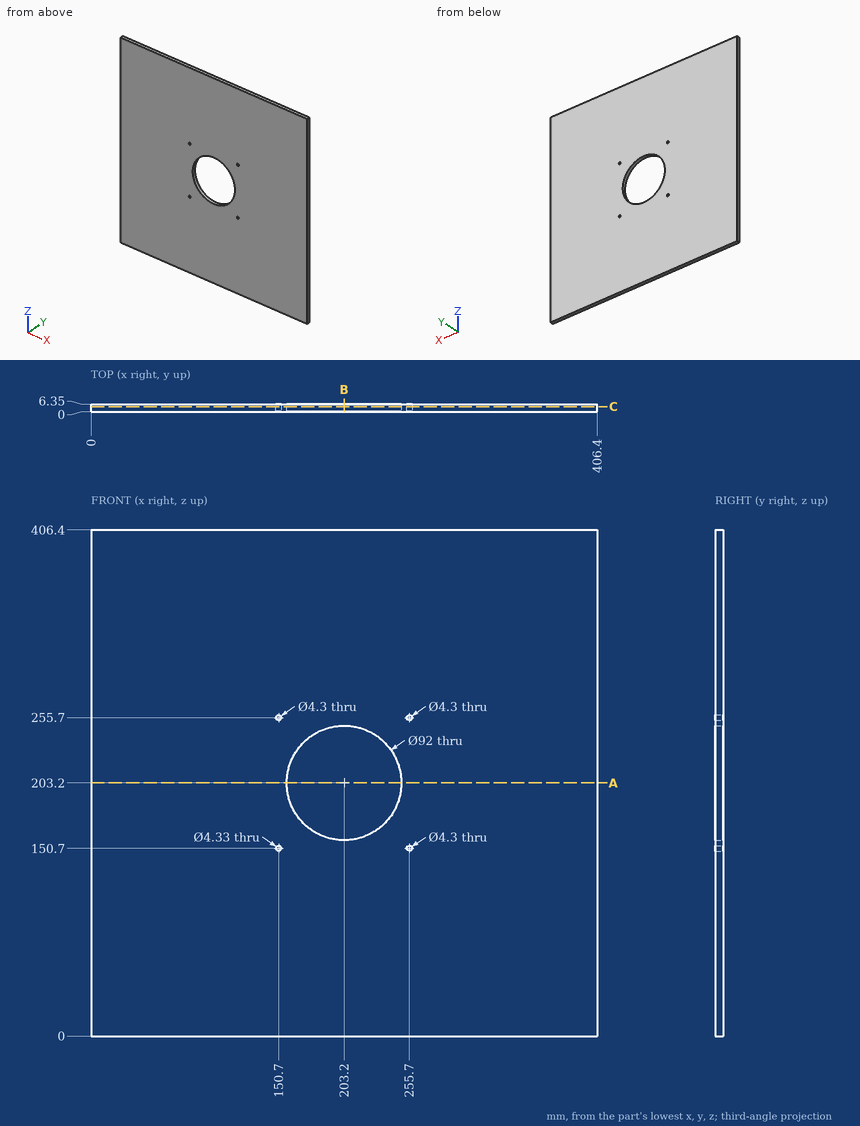
Input: dimensioned drawing with shaded views. Units: mm. Origin: part minimum x, y, z. Give positions to 0.01 mm unless a question says otherwise; leave off trailing zeros. Write each loop counter-clockwise with the first axis right and the second up, starting at its lowest first coordinate (ties: lowest second). Pieces come first, ordered by that corner, then holes. Notation, with made-up numbers: (56.25, -14.75) - (73.25, -14.75) arc R15 ccw to (73.25, 4.25) - close; hole circle Ø5 at (-19, -7). An arc over 180 degrees is marked (long way). One line per item, written item: value. Start each with the question number.
Q1. First-contact query: pin 1 Ø7 at (x, z) = (150.7, 255.7) entering from +Y. Flat tip, straight axial feed; report the tip coordinate or a pass-through.
Q2. Section query C-C, the plane y = 4.25. Return the cut outline in (x, z) (3 decimals), then the cut area to 3 significant figures.
Q3. Section query B-B, the plane x = 203.2. Return the cut outline in (y, z).
Q4. Material intervals for probe 1 along X at (y, z) = (1.75, 255.7); probe 2 along X at (y, z) = (3.5, 150.7) (3 decimals), sorted ascending. Write a range as from..to.
Q5. Section query A-A, the plane z = 203.2. Return the cut outline in (x, y).
Answer:
1. pin 1: stops at y = 6.35
2. outline: (0, 0) - (406.4, 0) - (406.4, 406.4) - (0, 406.4) - close; hole circle Ø4.33 at (150.7, 150.7); hole circle Ø4.3 at (150.7, 255.7); hole circle Ø92 at (203.2, 203.2); hole circle Ø4.3 at (255.7, 150.7); hole circle Ø4.3 at (255.7, 255.7)
2. area: 158,000 mm2
3. outline: (0, 0) - (6.35, 0) - (6.35, 157.2) - (0, 157.2) - close; (0, 249.2) - (6.35, 249.2) - (6.35, 406.4) - (0, 406.4) - close
4. probe 1: x = 0..148.55, 152.85..253.55, 257.85..406.4
4. probe 2: x = 0..148.535, 152.865..253.55, 257.85..406.4
5. outline: (0, 0) - (157.2, 0) - (157.2, 6.35) - (0, 6.35) - close; (249.2, 0) - (406.4, 0) - (406.4, 6.35) - (249.2, 6.35) - close
